```python
from build123d import *

# Parameters (mm, degrees)
SKETCH1_R                 = 0.8
BOSS_EXTRUDE2_DEPTH       = 2.4
BOSS_EXTRUDE4_DEPTH       = 34.2
BOSS_EXTRUDE7_OUTLINE_R   = 0.8
BOSS_EXTRUDE7_DEPTH       = 37.2
SKETCH1_10_R              = 0.8
CUT_EXTRUDE6_DEPTH        = 34.2
SKETCH1_11_R              = 0.8
BOSS_EXTRUDE8_DEPTH       = 2
BOSS_EXTRUDE9_START       = -49.8
BOSS_EXTRUDE9_OUTLINE_W   = 8.2
BOSS_EXTRUDE9_OUTLINE_H   = 10
BOSS_EXTRUDE9_OUTLINE_R   = 2.5
BOSS_EXTRUDE9_OUTLINE_H_2 = 4
BOSS_EXTRUDE9_DEPTH       = 49.8
BOSS_EXTRUDE10_START      = -44.4
SKETCH9_3_R               = 2.5
BOSS_EXTRUDE10_DEPTH      = 44.4
CUT_EXTRUDE7_START        = -5.4
SKETCH9_4_R               = 2.5
CUT_EXTRUDE7_DEPTH        = 5.4
CUT_EXTRUDE8_START        = -37.2
CUT_EXTRUDE8_DEPTH        = 37.2
BOSS_EXTRUDE12_START      = -3
BOSS_EXTRUDE12_DEPTH      = 3


# Read off the part's stored shape, not the designer's step: Boss-Extrude7, Boss-Extrude9
with BuildPart() as part:
    # Sketch1 → Boss-Extrude2 (new body)
    with BuildSketch(Plane(origin=(0, 0, 0), x_dir=(1, 0, 0), z_dir=(0, 1, 0))):
        Polygon((-10.4, 16.242178951), (-10.4, 30.95), (-16.8, 30.95), (-16.8, -18.85), (16.8, -18.85), (16.8, 30.95), (10.4, 30.95), (10.4, 16.242178951), (7.2, 13.042178951), (7.2, -14.85), (-7.2, -14.85), (-7.2, 13.042178951), align=None)
        with Locations(Location((-10.25, -8.45, 0), (0, 0, 270))):
            Circle(SKETCH1_R, mode=Mode.SUBTRACT)
        with Locations(Location((-10.25, 12.25, 0), (0, 0, 270))):
            Circle(SKETCH1_R, mode=Mode.SUBTRACT)
        with Locations(Location((-10.25, -12.25, 0), (0, 0, 270))):
            Circle(SKETCH1_R, mode=Mode.SUBTRACT)
        with Locations(Location((10.25, -8.45, 0), (0, 0, 270))):
            Circle(SKETCH1_R, mode=Mode.SUBTRACT)
        with Locations(Location((10.25, -12.25, 0), (0, 0, 270))):
            Circle(SKETCH1_R, mode=Mode.SUBTRACT)
        with Locations(Location((10.25, 12.25, 0), (0, 0, 270))):
            Circle(SKETCH1_R, mode=Mode.SUBTRACT)
    extrude(amount=BOSS_EXTRUDE2_DEPTH)

    # Sketch1<6> → Boss-Extrude4 (add)
    with BuildSketch(Plane(origin=(0, 0, 0), x_dir=(1, 0, 0), z_dir=(0, 1, 0))):
        Polygon((-12.8, -14.85), (-12.8, 30.95), (-16.8, 30.95), (-16.8, -18.85), (16.8, -18.85), (16.8, 30.95), (12.8, 30.95), (12.8, -14.85), align=None)
    extrude(amount=BOSS_EXTRUDE4_DEPTH)

    # Boss-Extrude7 outline → Boss-Extrude7 (add)
    with BuildSketch(Plane(origin=(0, 0, 0), x_dir=(1, 0, 0), z_dir=(0, 1, 0))):
        Polygon((16.8, -18.85), (16.8, 30.95), (10.4, 30.95), (10.4, 16.242178951), (9.4, 15.242178951), (9.4, 9.2), (10.3, 9.2), (10.3, 3.8), (9.4, 3.8), (9.4, -9.55), (-9.4, -9.55), (-9.4, 3.9), (-10.3, 3.9), (-10.3, 9.2), (-9.4, 9.2), (-9.4, 15.242178951), (-10.4, 16.242178951), (-10.4, 30.95), (-16.8, 30.95), (-16.8, -18.85), align=None)
        with Locations((-10.25, 12.25)):
            Circle(BOSS_EXTRUDE7_OUTLINE_R, mode=Mode.SUBTRACT)
        with Locations((-10.25, -12.25)):
            Circle(BOSS_EXTRUDE7_OUTLINE_R, mode=Mode.SUBTRACT)
        with Locations((10.25, 12.25)):
            Circle(BOSS_EXTRUDE7_OUTLINE_R, mode=Mode.SUBTRACT)
        with Locations((10.25, -12.25)):
            Circle(BOSS_EXTRUDE7_OUTLINE_R, mode=Mode.SUBTRACT)
    extrude(amount=BOSS_EXTRUDE7_DEPTH)

    # Sketch1<10> → Cut-Extrude6 (cut)
    with BuildSketch(Plane(origin=(0, 0, 0), x_dir=(1, 0, 0), z_dir=(0, 1, 0))):
        Polygon((-10.4, 16.242178951), (-10.4, 30.95), (-12.8, 30.95), (-12.8, -14.85), (12.8, -14.85), (12.8, 30.95), (10.4, 30.95), (10.4, 16.242178951), (7.2, 13.042178951), (7.2, -9.55), (-7.2, -9.55), (-7.2, 13.042178951), align=None)
        with Locations(Location((-10.25, 12.25, 0), (0, 0, 270))):
            Circle(SKETCH1_10_R, mode=Mode.SUBTRACT)
        with Locations(Location((-10.25, -12.25, 0), (0, 0, 270))):
            Circle(SKETCH1_10_R, mode=Mode.SUBTRACT)
        with Locations(Location((10.25, -12.25, 0), (0, 0, 270))):
            Circle(SKETCH1_10_R, mode=Mode.SUBTRACT)
        with Locations(Location((10.25, 12.25, 0), (0, 0, 270))):
            Circle(SKETCH1_10_R, mode=Mode.SUBTRACT)
    extrude(amount=CUT_EXTRUDE6_DEPTH, mode=Mode.SUBTRACT)

    # Sketch1<11> → Boss-Extrude8 (add)
    # profile 1 of 2: a face of its own
    with BuildSketch(Plane(origin=(0, 0, 0), x_dir=(1, 0, 0), z_dir=(0, 1, 0))):
        Polygon((-10.4, 16.242178951), (-10.4, 30.95), (-12.8, 30.95), (-12.8, -14.85), (-7.2, -14.85), (-7.2, 13.042178951), align=None)
        with Locations(Location((-10.25, -8.45, 0), (0, 0, 270))):
            Circle(SKETCH1_11_R, mode=Mode.SUBTRACT)
        with Locations(Location((-10.25, 12.25, 0), (0, 0, 270))):
            Circle(SKETCH1_11_R, mode=Mode.SUBTRACT)
    # profile 2 of 2: a face of its own
    with BuildSketch(Plane(origin=(0, 0, 0), x_dir=(1, 0, 0), z_dir=(0, 1, 0))):
        Polygon((7.2, -14.85), (12.8, -14.85), (12.8, 30.95), (10.4, 30.95), (10.4, 16.242178951), (7.2, 13.042178951), align=None)
        with Locations(Location((10.25, -8.45, 0), (0, 0, 270))):
            Circle(SKETCH1_11_R, mode=Mode.SUBTRACT)
        with Locations(Location((10.25, 12.25, 0), (0, 0, 270))):
            Circle(SKETCH1_11_R, mode=Mode.SUBTRACT)
    extrude(amount=BOSS_EXTRUDE8_DEPTH)

    # Boss-Extrude9 outline → Boss-Extrude9 (add)
    # profile 1 of 6: a face of its own
    with BuildSketch(Plane.XY.offset(18.85).offset(BOSS_EXTRUDE9_START)):
        with Locations((20.9, 5)):
            Rectangle(BOSS_EXTRUDE9_OUTLINE_W, BOSS_EXTRUDE9_OUTLINE_H)
        with Locations((20, 5)):
            Circle(BOSS_EXTRUDE9_OUTLINE_R, mode=Mode.SUBTRACT)
    # profile 2 of 6: a face of its own
    with BuildSketch(Plane.XY.offset(18.85).offset(BOSS_EXTRUDE9_START)):
        with Locations((-20.9, 5)):
            Rectangle(BOSS_EXTRUDE9_OUTLINE_W, BOSS_EXTRUDE9_OUTLINE_H)
        with Locations((-20, 5)):
            Circle(BOSS_EXTRUDE9_OUTLINE_R, mode=Mode.SUBTRACT)
    # profile 3 of 6: a face of its own
    with BuildSketch(Plane.XY.offset(18.85).offset(BOSS_EXTRUDE9_START)):
        with Locations((20.9, 25)):
            Rectangle(BOSS_EXTRUDE9_OUTLINE_W, BOSS_EXTRUDE9_OUTLINE_H)
        with Locations((20, 25)):
            Circle(BOSS_EXTRUDE9_OUTLINE_R, mode=Mode.SUBTRACT)
    # profile 4 of 6: a face of its own
    with BuildSketch(Plane.XY.offset(18.85).offset(BOSS_EXTRUDE9_START)):
        with Locations((-20.9, 25)):
            Rectangle(BOSS_EXTRUDE9_OUTLINE_W, BOSS_EXTRUDE9_OUTLINE_H)
        with Locations((-20, 25)):
            Circle(BOSS_EXTRUDE9_OUTLINE_R, mode=Mode.SUBTRACT)
    # profile 5 of 6: a face of its own
    with BuildSketch(Plane.XY.offset(18.85).offset(BOSS_EXTRUDE9_START)):
        with Locations((20.9, 35.2)):
            Rectangle(BOSS_EXTRUDE9_OUTLINE_W, BOSS_EXTRUDE9_OUTLINE_H_2)
    # profile 6 of 6: a face of its own
    with BuildSketch(Plane.XY.offset(18.85).offset(BOSS_EXTRUDE9_START)):
        with Locations((-20.9, 35.2)):
            Rectangle(BOSS_EXTRUDE9_OUTLINE_W, BOSS_EXTRUDE9_OUTLINE_H_2)
    extrude(amount=BOSS_EXTRUDE9_DEPTH)

    # Sketch9<3> → Boss-Extrude10 (add)
    with BuildSketch(Plane.XY.offset(18.85).offset(BOSS_EXTRUDE10_START)):
        with Locations((-20, 25)):
            Circle(SKETCH9_3_R)
        with Locations((-20, 5)):
            Circle(SKETCH9_3_R)
        with Locations((20, 5)):
            Circle(SKETCH9_3_R)
        with Locations((20, 25)):
            Circle(SKETCH9_3_R)
    extrude(amount=BOSS_EXTRUDE10_DEPTH)

    # Sketch9<4> → Cut-Extrude7 (cut)
    with BuildSketch(Plane.XY.offset(18.85).offset(CUT_EXTRUDE7_START)):
        with Locations((-20, 25)):
            Circle(SKETCH9_4_R)
        with Locations((-20, 5)):
            Circle(SKETCH9_4_R)
        with Locations((20, 5)):
            Circle(SKETCH9_4_R)
        with Locations((20, 25)):
            Circle(SKETCH9_4_R)
    extrude(amount=CUT_EXTRUDE7_DEPTH, mode=Mode.SUBTRACT)

    # Sketch12 → Cut-Extrude8 (cut)
    with BuildSketch(Plane(origin=(0, 37.2, 0), x_dir=(1, 0, 0), z_dir=(0, 1, 0)).offset(CUT_EXTRUDE8_START)):
        Polygon((-16.8, 13.896914247), (-25, 22.096914247), (-25, -9.996914247), (-16.8, -1.796914247), align=None)
        Polygon((16.8, -1.796914247), (25, -9.996914247), (25, 22.096914247), (16.8, 13.896914247), align=None)
    extrude(amount=CUT_EXTRUDE8_DEPTH, mode=Mode.SUBTRACT)

    # Sketch14 → Boss-Extrude12 (add)
    with BuildSketch(Plane(origin=(0, 37.2, 0), x_dir=(1, 0, 0), z_dir=(0, 1, 0)).offset(BOSS_EXTRUDE12_START)):
        with BuildLine():
            ThreePointArc((-10.3, 13.048435971), (-11.05, 12.25), (-10.3, 11.451564029))
            Line((-10.3, 11.451564029), (-10.3, 13.048435971))
        make_face()
        with BuildLine():
            Line((-10.3, 13.048435971), (-10.3, 11.451564029))
            ThreePointArc((-10.3, 11.451564029), (-9.702277442, 11.666904811), (-9.45, 12.25))
            ThreePointArc((-9.45, 12.25), (-9.702277442, 12.833095189), (-10.3, 13.048435971))
        make_face()
        with BuildLine():
            ThreePointArc((10.3, 13.048435971), (9.45, 12.25), (10.3, 11.451564029))
            Line((10.3, 11.451564029), (10.3, 13.048435971))
        make_face()
        with BuildLine():
            Line((10.3, 13.048435971), (10.3, 11.451564029))
            ThreePointArc((10.3, 11.451564029), (10.833095189, 11.702277442), (11.05, 12.25))
            ThreePointArc((11.05, 12.25), (10.833095189, 12.797722558), (10.3, 13.048435971))
        make_face()
    extrude(amount=BOSS_EXTRUDE12_DEPTH)


solid = part.part
```
Geometry check sheet. Reference: the model listing, model coordinates, mm. A direction names the side the tool comes from. Round coordinates to 2 decimals unless told otherwise and drop trailing zeros. Order: outer loops, then holes, each group sorted by start corner. A loop starts at its lowest first (then second) coordinate and runs counter-clockwise, first axis right, second up. Notation, with made-up numbers: (27, 8) -> (55, 8) arc R10 cw to (55, 26) -> close; hole circle Ø8 at (69.5, 55.5). An arc over 180 degrees is marked (long way). Return JSON: item names as keys, results as strings. Group by question number.
Q1. Tool access check on faces 1 (the flat face through (0, 17, 14.85)), 2 (the flat face through (16.8, 18, -6)), 3 (the flat face through (-21, 33.2, -24)), 4 (the cylindrical face through (-22.5, 5.1, 16.1)). Record the directions out of +Z, -Z, +X, -X, +Y, -Y that give a thin tool (end or side, any length) a straight path to the whole face; none if there is none.
Q2. Section check A-A, the plane z = -12.25. Record the boundary of the cut face in (x, y), plus the area to 3 significant figures.
Q3. Section check D-D, the plane z = 12.25. Count the separate pieces of the cut face and the enclosed holes in it, plus the area to 3 significant figures.
Q4. Material ranges on probe 1 along Y at (x, z) = (-17, -24.5); probe 2 along X at (y, z) = (0.65, -12.25); probe 3 along Y at (x, z) = (-20, -28.05), recorded low to high. Write a range as from..to.
Q5. Gauge pin test, flat ends, axial feed: pin 1 (2.5 mm diameter, centred on y = 36, z = -11, fed in from -X); pin 2 (1.5 mm diameter, centred on x = -21, y = 5.5, fed in from -Z); pin 3 (3 mm diameter, centred on x = 20, y = 5, fed in from +Z). Record the tip position at first contact, or that the pin passes through.
Q6. Release check for a two-part mould opening along Y. For faces 5 (the flat face through (-20.843, 4.93, -17.94)), 6 (the flat face through (21, 33.2, 12)), 7 (the flat face through (20, 25, -25.55)), 8 (the flat face through (11, 37.2, -6)) record: released by +Y, released by -Y, zero draft, split by the parting line, or undercut.
Numbers:
{
 "1": {"face 1": "-Z", "face 2": "+X", "face 3": "+Z, -Z, -X", "face 4": "+Z"},
 "2": {"outline": "(-16.8, 0) -> (-11.05, 0) -> (-11.05, 2) -> (-12.8, 2) -> (-12.8, 34.2) -> (-9.4, 34.2) -> (-9.4, 37.2) -> (-16.8, 37.2) -> close; (-9.45, 0) -> (-7.2, 0) -> (-7.2, 2) -> (-9.45, 2) -> close; (7.2, 0) -> (9.45, 0) -> (9.45, 2) -> (7.2, 2) -> close; (9.4, 34.2) -> (12.8, 34.2) -> (12.8, 2) -> (11.05, 2) -> (11.05, 0) -> (16.8, 0) -> (16.8, 37.2) -> (9.4, 37.2) -> close", "area": "334 mm^2"},
 "3": {"separate pieces": "3", "enclosed holes": "0", "area": "781 mm^2"},
 "4": {"probe 1": "0..10, 20..30, 33.2..37.2", "probe 2": "-16.8..-11.05, -9.45..-7.2, 7.2..9.45, 11.05..16.8", "probe 3": "0..2.5, 7.5..10, 20..22.5, 27.5..30, 33.2..37.2"},
 "5": {"pin 1": "x = -16.8", "pin 2": "z = -25.55", "pin 3": "z = 13.45"},
 "6": {"face 5": "zero draft", "face 6": "undercut", "face 7": "undercut", "face 8": "released by +Y"}
}
